The listing builds one solid part. Answer for the finished solid, in the listing's coordinates (mm). A direction names the side the tool comes from. Give positions to 0.01 mm unless a question says otherwise; leave off trailing zeros. Order: outer loops, then holes, each group sorted by start corner. A loop starts at its lowest first (then second) coordinate and runs counter-clockwise, first axis right, second up. Notation, with made-up numbers: (-30.75, -5) - (-9.75, -5) arc R15 ccw to (-9.75, 10) - close; hole circle Ø9 at (77, 33). An arc over 180 degrees is marked (long way). Answer in a Markdown table with one row per item.
from build123d import *

# Parameters (mm, degrees)
F0_W      = 60
F0_H      = 13
F1_DEPTH  = 42
F2_T      = -0.5
F3_W      = 32
F3_H      = 10
F4_DEPTH  = 25
F5_W      = 17
F5_H      = 40
F6_DEPTH  = 25
F7_R      = 3.5
F8_DEPTH  = 30
F9_T      = -1
F10_R     = 3.5
F11_DEPTH = 25


with BuildPart() as f1:
    # F0 (on Front) → F1 (new body)
    with BuildSketch(Plane.XZ):
        with Locations((30, 6.5)):
            Rectangle(F0_W, F0_H)
    extrude(amount=F1_DEPTH)

    # F2
    f2_openings = [f1.faces().sort_by_distance(p)[0] for p in [
        (0, -21, 6.5),
    ]]
    offset(amount=F2_T, openings=f2_openings)

    # F3 (on face) → F4 (cut)
    with BuildSketch(Plane.YZ.offset(60)):
        with Locations((-21, 5.9)):
            Rectangle(F3_W, F3_H)
    extrude(amount=-F4_DEPTH, mode=Mode.SUBTRACT)

    # F5 (on face) → F6 (cut)
    with BuildSketch(Plane.XY.offset(13)):
        with Locations((14.4643624128, -21)):
            Rectangle(F5_W, F5_H)
        with Locations((45.5356375872, -21)):
            Rectangle(F5_W, F5_H)
    extrude(amount=-F6_DEPTH, mode=Mode.SUBTRACT)

    # F7 (on face) → F8 (join)
    with BuildSketch(Plane(origin=(0, 0, 0), x_dir=(-1, 0, 0), z_dir=(0, 1, 0))):
        with Locations((-30, 6.5)):
            Circle(F7_R)
    extrude(amount=F8_DEPTH)

    # F9
    f9_openings = [f1.faces().sort_by_distance(p)[0] for p in [
        (30, 30, 6.5),
    ]]
    offset(amount=F9_T, openings=f9_openings)

    # F10 (on face) → F11 (join)
    with BuildSketch(Plane(origin=(0, 0, 0), x_dir=(-1, 0, 0), z_dir=(0, 1, 0))):
        with BuildLine():
            Line((-34.4180972565, 6.3872897981), (-34.4180972565, 6.6127102019))
            ThreePointArc((-34.4180972565, 6.6127102019), (-34.4195346992, 6.5), (-34.4180972565, 6.3872897981))
        make_face()
        with BuildLine():
            ThreePointArc((-34.4180972565, 6.3872897981), (-29.9436403161, 2.0808246761), (-25.5804653008, 6.5))
            ThreePointArc((-25.5804653008, 6.5), (-29.9436403161, 10.9191753239), (-34.4180972565, 6.6127102019))
            Line((-34.4180972565, 6.6127102019), (-34.4180972565, 6.3872897981))
        make_face()
        with Locations((-30, 6.5)):
            Circle(F10_R, mode=Mode.SUBTRACT)
        with BuildLine():
            ThreePointArc((-34.4180972565, 6.3872897981), (-34.4195346992, 6.5), (-34.4180972565, 6.6127102019))
            Line((-34.4180972565, 6.6127102019), (-35.146126033, 6.6127102019))
            Line((-35.146126033, 6.6127102019), (-35.146126033, 6.3872897981))
            Line((-35.146126033, 6.3872897981), (-34.4180972565, 6.3872897981))
        make_face()
    extrude(amount=F11_DEPTH)


solid = f1.part
Item 1: Determine the mould class of faces 1 (the face through (34, 25, 6)), 2 (the face through (32.5, 15, 6.6)), 3 (the face through (29, -21, 12.5)), 4 (the face through (29, -41.5, 7)) for opening direction Y: pulls with the +Y half, pulls with the -Y half, needs draft (parallel to the pull), parting line crosses it, or undercut.
Answer block:
| item | result |
|---|---|
| face 1 | pulls with the +Y half |
| face 2 | needs draft |
| face 3 | undercut |
| face 4 | undercut |
Item 2: Find section B-B on y = -18. Write down the section's boundary in (x, z), then the cut area to 3 significant figures.
Answer block:
| item | result |
|---|---|
| outline | (0, 0) - (5.96, 0) - (5.96, 0.5) - (0, 0.5) - close; (0, 12.5) - (5.96, 12.5) - (5.96, 13) - (0, 13) - close; (22.96, 0) - (37.04, 0) - (37.04, 0.5) - (22.96, 0.5) - close; (22.96, 12.5) - (37.04, 12.5) - (37.04, 13) - (22.96, 13) - close; (54.04, 0) - (60, 0) - (60, 0.9) - (59.5, 0.9) - (59.5, 0.5) - (54.04, 0.5) - close; (54.04, 12.5) - (59.5, 12.5) - (59.5, 10.9) - (60, 10.9) - (60, 13) - (54.04, 13) - close |
| area | 27.0 mm² |
Item 3: Find section A-A on x = 30. Write down the section's boundary in (y, z).
Answer block:
| item | result |
|---|---|
| outline | (-42, 0) - (0, 0) - (0, 2.08) - (25, 2.08) - (25, 3) - (30, 3) - (30, 4) - (0.5, 4) - (0.5, 9) - (30, 9) - (30, 10) - (25, 10) - (25, 10.92) - (0, 10.92) - (0, 13) - (-42, 13) - close; hole (-41.5, 0.5) - (-0.5, 0.5) - (-0.5, 12.5) - (-41.5, 12.5) - close |
Item 4: Consider line 1 (Y direction, x = 13, z = 5.25); line 2 (Z direction, x = 30, y = 19); line 3 (Z direction, x = 36, y = -30). Determine where each line is inside the solid, lowest interval first.
Answer block:
| item | result |
|---|---|
| line 1 | -42 to -41.5, -0.5 to 0 |
| line 2 | 2.08 to 4, 9 to 10.92 |
| line 3 | 0 to 0.5, 12.5 to 13 |
Item 5: Each of these flat-tipped pins is pushed along its axis until it touches: P1, Ø8, axis at x = 30, y = -28.5, coming from the -Z side; P2, Ø1, axis at y = 21.5, z = 2, coming from the -X side; P3, Ø0.6, axis at x = 13, z = 0.5, coming from the +Y side; P4, Ø4, axis at x = 29, y = 19, coming from the +Z side. Where does it stop, or does it pass through?
Answer block:
| item | result |
|---|---|
| P1 | z = 0 |
| P2 | x = 28.12 |
| P3 | y = 0 |
| P4 | z = 10.92 |
Item 6: Find section D-D on y = 21.5. Write down the section's boundary in (x, z).
Answer block:
| item | result |
|---|---|
| outline | (34.42, 6.39) - (35.15, 6.39) - (35.15, 6.61) - (34.42, 6.61) arc R4.42 ccw (long way) to start; hole circle Ø5 at (30, 6.5) |
Item 7: Find section C-C on x = 52. Write down the section's boundary in (y, z).
Answer block:
| item | result |
|---|---|
| outline | (-42, 0) - (-41, 0) - (-41, 0.5) - (-41.5, 0.5) - (-41.5, 12.5) - (-41, 12.5) - (-41, 13) - (-42, 13) - close; (-1, 0) - (0, 0) - (0, 13) - (-1, 13) - (-1, 12.5) - (-0.5, 12.5) - (-0.5, 0.5) - (-1, 0.5) - close |
Item 8: Which of the six approach directions +Z, -Z, +X, -X, +Y, -Y give full straight-line access (tool end or side, diameter ignored) to faces 5 (the face through (60, -20.7, 0.6)), 6 (the face through (29, -21, 0.5)), 7 (the face through (26.767, 27.465, 5.159))?
Answer block:
| item | result |
|---|---|
| face 5 | +Z, -Z, +X, +Y, -Y |
| face 6 | -X |
| face 7 | +Y |
